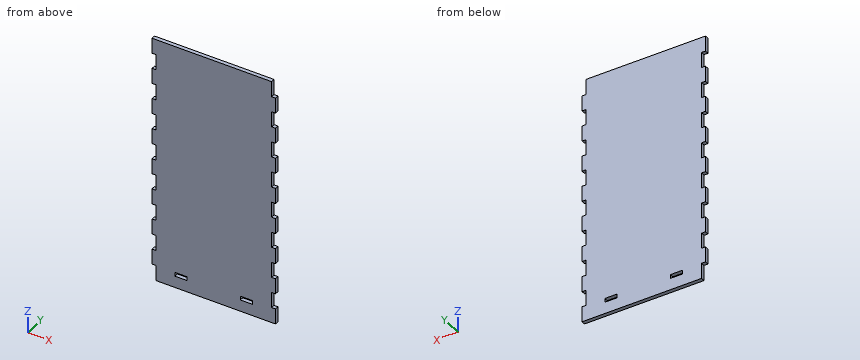
Autodesk Fusion 360 part; units mm, degrees
sketch "Sketch1" plane through (0, 0, 0) normal (0, 1, 0) x (1, 0, 0)
  line L0 (3.175, -50.8) -> (3.175, -38.1)
  line L1 (3.175, -38.1) -> (3.175, -25.4)
  line L2 (6.35, -12.7) -> (3.175, -12.7)
  line L3 (3.175, -63.5) -> (6.35, -63.5)
  line L4 (3.175, -76.2) -> (3.175, -63.5)
  line L5 (6.35, -25.4) -> (3.175, -25.4)
  line L6 (3.175, -88.9) -> (3.175, -76.2)
  line L7 (6.35, -25.4) -> (6.35, -38.1)
  line L8 (6.35, -38.1) -> (3.175, -38.1)
  line L9 (3.175, -12.7) -> (3.175, 0)
  line L10 (3.175, -60.2676) -> (2.1543, -60.2676)
  line L11 (3.175, 0) -> (3.175, -59.055)
  line L12 (6.35, 0) -> (3.175, 0)
  line L13 (3.175, -25.4) -> (3.175, -12.7)
  line L14 (3.175, -101.6) -> (3.175, -88.9)
  line L15 (3.175, -76.2) -> (6.35, -76.2)
  line L16 (-95.25, -25.4) -> (-95.25, -12.7)
  line L17 (-92.075, -139.7) -> (-95.25, -139.7)
  line L18 (3.175, 0) -> (3.175, -203.2)
  line L19 (-92.075, -50.8) -> (-95.25, -50.8)
  line L20 (3.175, -50.8) -> (6.35, -50.8)
  line L21 (6.35, 0) -> (-4.7498, 0)
  line L22 (3.175, -88.9) -> (6.35, -88.9)
  line L23 (-92.075, -38.1) -> (-92.075, -25.4)
  line L24 (-92.075, -127) -> (-92.075, -114.3)
  line L25 (-95.25, 0) -> (6.35, 0)
  line L26 (-92.075, -203.2) -> (-92.075, -190.5)
  line L27 (3.175, -63.5) -> (3.175, -50.8)
  line L28 (6.35, -50.8) -> (6.35, -63.5)
  line L29 (-92.075, 0) -> (-92.075, -203.2)
  line L30 (6.35, -76.2) -> (6.35, -88.9)
  line L31 (-92.075, -95.25) -> (-92.075, -88.9)
  line L32 (6.35, 0) -> (-5.715, 0)
  line L33 (-95.25, 0) -> (-79.375, 0)
  line L34 (-92.075, -25.4) -> (-95.25, -25.4)
  line L35 (-92.075, -76.2) -> (-92.075, -63.5)
  line L36 (-4.7498, 0) -> (0.3302, 0)
  line L37 (6.35, 0) -> (6.35, -12.7)
  line L38 (6.35, -101.6) -> (3.175, -101.6)
  line L39 (-92.075, -177.8) -> (-95.25, -177.8)
  line L40 (-84.1502, 0) -> (-89.2302, 0)
  line L41 (-92.075, -139.7) -> (-92.075, -127)
  line L42 (-89.5189, -92.8088) -> (-89.7576, -92.8956)
  line L43 (-95.25, -101.6) -> (-95.25, -88.9)
  line L44 (6.35, -177.8) -> (6.35, -190.5)
  line L45 (6.35, -152.4) -> (6.35, -165.1)
  line L46 (3.175, -203.2) -> (3.175, -190.5)
  line L47 (3.175, -190.5) -> (3.175, -177.8)
  line L48 (-92.075, -63.5) -> (-95.25, -63.5)
  line L49 (-92.075, -25.4) -> (-92.075, -12.7)
  line L50 (-92.075, -190.5) -> (-95.25, -190.5)
  line L51 (-92.075, -12.7) -> (-95.25, -12.7)
  line L52 (3.175, -203.2) -> (-95.25, -203.2)
  line L53 (-92.075, -177.8) -> (-92.075, -165.1)
  line L54 (-92.075, -101.6) -> (-92.075, -95.25)
  line L55 (-92.075, -76.2) -> (-95.25, -76.2)
  line L56 (-95.25, -76.2) -> (-95.25, -63.5)
  line L57 (3.175, -114.3) -> (6.35, -114.3)
  line L58 (-95.25, -203.2) -> (-95.25, -190.5)
  line L59 (-92.075, -63.5) -> (-92.075, -50.8)
  line L60 (-92.075, -50.8) -> (-92.075, -38.1)
  line L61 (-92.075, -152.4) -> (-95.25, -152.4)
  line L62 (-92.075, -88.9) -> (-95.25, -88.9)
  line L63 (-92.075, -152.4) -> (-92.075, -139.7)
  line L64 (-95.25, -203.2) -> (-92.075, -203.2)
  line L65 (6.35, -152.4) -> (3.175, -152.4)
  line L66 (-92.075, -165.1) -> (-92.075, -152.4)
  line L67 (-92.075, -203.2) -> (-92.075, -177.8)
  line L68 (-92.075, -165.1) -> (-95.25, -165.1)
  line L69 (-92.075, -114.3) -> (-95.25, -114.3)
  line L70 (6.35, -101.6) -> (6.35, -114.3)
  line L71 (-95.25, -127) -> (-95.25, -114.3)
  line L72 (-92.075, -114.3) -> (-92.075, -101.6)
  line L73 (6.35, -139.7) -> (6.35, -127)
  line L74 (6.35, -127) -> (6.35, -139.7)
  line L75 (3.175, -177.8) -> (6.35, -177.8)
  line L76 (3.175, -165.1) -> (6.35, -165.1)
  line L77 (-92.075, -38.1) -> (-95.25, -38.1)
  line L78 (6.35, -114.3) -> (6.35, -101.6)
  line L79 (-95.25, 0) -> (-84.1502, 0)
  line L80 (-92.075, -127) -> (-95.25, -127)
  line L81 (3.175, -152.4) -> (3.175, -139.7)
  line L82 (-95.25, -177.8) -> (-95.25, -165.1)
  line L83 (6.35, -165.1) -> (6.35, -152.4)
  line L84 (-92.075, -101.6) -> (-95.25, -101.6)
  line L85 (3.175, -139.7) -> (6.35, -139.7)
  line L86 (-95.25, 0) -> (-92.075, 0)
  line L87 (-95.25, -152.4) -> (-95.25, -139.7)
  line L88 (3.175, -127) -> (3.175, -114.3)
  line L89 (6.35, -127) -> (3.175, -127)
  line L90 (3.175, -190.5) -> (6.35, -190.5)
  line L91 (-92.075, -88.9) -> (-92.075, -76.2)
  line L92 (-95.25, 0) -> (-93.6625, 0)
  line L93 (-92.075, -190.5) -> (-92.075, -177.8)
  line L94 (3.175, -177.8) -> (3.175, -165.1)
  line L95 (-95.25, -50.8) -> (-95.25, -38.1)
  point P0 (6.35, 0)
  point P1 (6.35, 0)
  dimension "d9" = 11.0998
  dimension "d10" = 11.0998
  dimension "d14" = 5.08
  dimension "d15" = 5.08
  dimension "d27" = 3.175
  dimension "d28" = 3.175
  dimension "d40" = 3.175
  dimension "d41" = 3.175
  dimension "d42" = 12.7
  dimension "d43" = 12.7
  dimension "d44" = 12.7
  dimension "d45" = 12.7
  dimension "d46" = 12.7
  dimension "d47" = 12.7
  dimension "d48" = 12.7
  dimension "d49" = 12.7
  dimension "d50" = 6.35
  dimension "d52" = 12.7
  dimension "d53" = 12.7
  dimension "d54" = 12.7
  dimension "d55" = 12.7
  dimension "d56" = 12.7
  dimension "d57" = 12.7
extrude "Extrude1" add sketch "Sketch1" along normal blind 3.175
sketch "Sketch2" plane through (0, 0, 0) normal (0, -1, 0) x (1, 0, 0)
  line L0 (-95.25, 63.5) -> (-92.075, 63.5)
  line L1 (-92.075, 63.5) -> (-92.075, 50.8)
  line L2 (-92.075, 50.8) -> (-95.25, 50.8)
  line L3 (-95.25, 50.8) -> (-95.25, 38.1)
  line L4 (-95.25, 38.1) -> (-92.075, 38.1)
  line L5 (-92.075, 38.1) -> (-92.075, 25.4)
  line L6 (-92.075, 25.4) -> (-95.25, 25.4)
  line L7 (-95.25, 25.4) -> (-95.25, 12.7)
  line L8 (-95.25, 12.7) -> (-92.075, 12.7)
  line L9 (-92.075, 12.7) -> (-92.075, 0)
  line L10 (-92.075, 0) -> (6.35, 0)
  line L11 (6.35, 0) -> (6.35, 12.7)
  line L12 (6.35, 12.7) -> (3.175, 12.7)
  line L13 (3.175, 12.7) -> (3.175, 25.4)
  line L14 (3.175, 25.4) -> (6.35, 25.4)
  line L15 (6.35, 25.4) -> (6.35, 38.1)
  line L16 (6.35, 38.1) -> (3.175, 38.1)
  line L17 (3.175, 38.1) -> (3.175, 50.8)
  line L18 (3.175, 50.8) -> (6.35, 50.8)
  line L19 (6.35, 50.8) -> (6.35, 63.5)
  line L20 (6.35, 63.5) -> (3.175, 63.5)
  line L21 (3.175, 63.5) -> (3.175, 76.2)
  line L22 (3.175, 76.2) -> (6.35, 76.2)
  line L23 (6.35, 76.2) -> (6.35, 88.9)
  line L24 (6.35, 88.9) -> (3.175, 88.9)
  line L25 (3.175, 88.9) -> (3.175, 101.6)
  line L26 (3.175, 101.6) -> (6.35, 101.6)
  line L27 (6.35, 101.6) -> (6.35, 114.3)
  line L28 (6.35, 114.3) -> (3.175, 114.3)
  line L29 (3.175, 114.3) -> (3.175, 127)
  line L30 (3.175, 127) -> (6.35, 127)
  line L31 (6.35, 127) -> (6.35, 139.7)
  line L32 (6.35, 139.7) -> (3.175, 139.7)
  line L33 (3.175, 139.7) -> (3.175, 152.4)
  line L34 (3.175, 152.4) -> (6.35, 152.4)
  line L35 (6.35, 152.4) -> (6.35, 165.1)
  line L36 (6.35, 165.1) -> (3.175, 165.1)
  line L37 (3.175, 165.1) -> (3.175, 177.8)
  line L38 (3.175, 177.8) -> (6.35, 177.8)
  line L39 (6.35, 177.8) -> (6.35, 190.5)
  line L40 (6.35, 190.5) -> (3.175, 190.5)
  line L41 (3.175, 190.5) -> (3.175, 203.2)
  line L42 (3.175, 203.2) -> (-95.25, 203.2)
  line L43 (-95.25, 203.2) -> (-95.25, 190.5)
  line L44 (-95.25, 190.5) -> (-92.075, 190.5)
  line L45 (-92.075, 190.5) -> (-92.075, 177.8)
  line L46 (-92.075, 177.8) -> (-95.25, 177.8)
  line L47 (-95.25, 177.8) -> (-95.25, 165.1)
  line L48 (-95.25, 165.1) -> (-92.075, 165.1)
  line L49 (-92.075, 165.1) -> (-92.075, 152.4)
  line L50 (-92.075, 152.4) -> (-95.25, 152.4)
  line L51 (-95.25, 152.4) -> (-95.25, 139.7)
  line L52 (-95.25, 139.7) -> (-92.075, 139.7)
  line L53 (-92.075, 139.7) -> (-92.075, 127)
  line L54 (-92.075, 127) -> (-95.25, 127)
  line L55 (-95.25, 127) -> (-95.25, 114.3)
  line L56 (-95.25, 114.3) -> (-92.075, 114.3)
  line L57 (-92.075, 114.3) -> (-92.075, 101.6)
  line L58 (-92.075, 101.6) -> (-95.25, 101.6)
  line L59 (-95.25, 101.6) -> (-95.25, 88.9)
  line L60 (-95.25, 88.9) -> (-92.075, 88.9)
  line L61 (-92.075, 88.9) -> (-92.075, 76.2)
  line L62 (-92.075, 76.2) -> (-95.25, 76.2)
  line L63 (-95.25, 76.2) -> (-95.25, 63.5)
  line L64 (6.35, 0) -> (-12.3698, 0)
  line L65 (-12.3698, 0) -> (-12.3698, 9.525)
  line L66 (-92.075, 0) -> (-76.5302, 0)
  line L67 (-76.5302, 0) -> (-76.5302, 9.525)
  line L68 (-76.5302, 9.525) -> (-66.3702, 9.525)
  line L69 (-66.3702, 9.525) -> (-66.3702, 12.7)
  line L70 (-66.3702, 12.7) -> (-76.5302, 12.7)
  line L71 (-76.5302, 12.7) -> (-76.5302, 9.525)
  line L72 (-12.3698, 9.525) -> (-22.5298, 9.525)
  line L73 (-22.5298, 9.525) -> (-22.5298, 12.7)
  line L74 (-22.5298, 12.7) -> (-12.3698, 12.7)
  line L75 (-12.3698, 12.7) -> (-12.3698, 9.525)
  dimension "d105" = 18.7198
  dimension "d106" = 9.525
  dimension "d107" = 15.5448
  dimension "d108" = 9.525
  dimension "d109" = 10.16
  dimension "d110" = 3.175
  dimension "d111" = 10.16
  dimension "d112" = 10.16
  dimension "d113" = 10.16
extrude "Extrude2" cut sketch "Sketch2" against normal blind 20.32 contours L68 L69 L70 L71 | L72 L73 L74 L75
equation "d9 = 0.5 in - 0.063 in"
Work out the finished part from the listing and answer in its coordinate system (mm). Give positions to 0.01 mm unless a question says otherwise; leave off trailing zeros. Loops run counter-clockwise (first coordinate to the right, second up) from the corner with the lowest first, then second, coordinate; pieces in that order, holes last. Notation, with made-up numbers: (-14, -24.75) -> (44, -24.75) arc R22 ccw to (44, 6.25) -> close; hole circle Ø7 at (23, -32). An arc over 180 degrees is marked (long way). Use a Markdown table: item, result. Add a question column.
1. Find the intervals of material crossed by probe 1 along Z at (x, y) = (-71, 2.8) (3 decimals); probe 2 along X at (y, z) = (2.4, 48.5) (3 decimals); probe 3 along X at (y, z) = (1.95, 156) (3 decimals), in increasing order.
2. Section B-B on y = 2.65 is taken. State how many separate pieces and enclosed holes the cut face has, and give its area (3 significant figures).
3. Section C-C on z = 121 is taken. Determine the outline of the cut face in (x, y) (3 decimals), and give its area (4 significant figures).
4. Section A-A on x = -69 is taken. Determine the outline of the cut face in (y, z) (3 decimals).
5. Flat-ended cylindrical pins translate along their axes: pin 1 Ø1.5 at (y, z) = (2.5, 119.5) entering from +X (3 decimals); pin 2 Ø1.6 at (y, z) = (2, 11) entering from -X (3 decimals). Find the tip coordinate at first contact, or state that the pin passes through.
Results below:
| question | item | result |
|---|---|---|
| 1 | probe 1 | z = 0 to 9.525, 12.7 to 203.2 |
| 1 | probe 2 | x = -95.25 to 3.175 |
| 1 | probe 3 | x = -92.075 to 6.35 |
| 2 | separate pieces | 1 |
| 2 | enclosed holes | 2 |
| 2 | area | 19,900 mm^2 |
| 3 | outline | (-95.25, 0) -> (3.175, 0) -> (3.175, 3.175) -> (-95.25, 3.175) -> close |
| 3 | area | 312.5 mm^2 |
| 4 | outline | (0, 0) -> (3.175, 0) -> (3.175, 9.525) -> (0, 9.525) -> close; (0, 12.7) -> (3.175, 12.7) -> (3.175, 203.2) -> (0, 203.2) -> close |
| 5 | pin 1 | stops at x = 3.175 |
| 5 | pin 2 | stops at x = -92.075 |
